Design review of the part shown in the three views and the two pictorial views. Dimensions are in mm from the part's minimum x, y and z. Round coordinates to 2 decimals unless told otherwise and drop trailing zeros. Order: outer loops, then holes, each group sorted by start corner. A loop starts at its lowest first (then second) coordinate and runs counter-clockwise, first axis right, second up. Notation, with made-up numbers: (2.5, 80) - (32.5, 80) arc R10 ccw to (32.5, 91) - close; hole circle Ø10 at (41.5, -20). An arc over 180 degrees is marked (long way). One line per question, with ' | ' between items. Start each with the question number.
Item 1: Add section B-B on x = 18.5. State the section outline as (y, z) points.
Item 2: Add section C-C on y = 10.25. State the section outline as (x, z) points, and give its area (3 significant figures).
Item 3: Add section A-A on z = 11.75. State the section outline as (x, y) points, and give its area (3 significant figures).
Item 4: Insertion check: pin 1 Ø12 at (x, z) = (30, 3.5) entering from +Y; pin 2 Ø0.6 at (y, z) = (1.5, 14.5) entering from +X; pin 3 Ø0.6 at (y, z) = (1, 16.5) entering from -X. Each pin has a flat end and moves straight along its axis. Give the tip position at first contact, or say it passes through.
Item 5: For L1, parallel to X at y = 1, z = 17; L2, parallel to Y at x = 25.5, z = 27; L3, parallel to Y at x = 36.5, z = 11, list the stretches that pass through material, from the lowest coordinate up. Write a range as [from, to].
Item 6: Add section D-D on y = 5. State the section outline as (x, z) points, and give its area (3 significant figures).
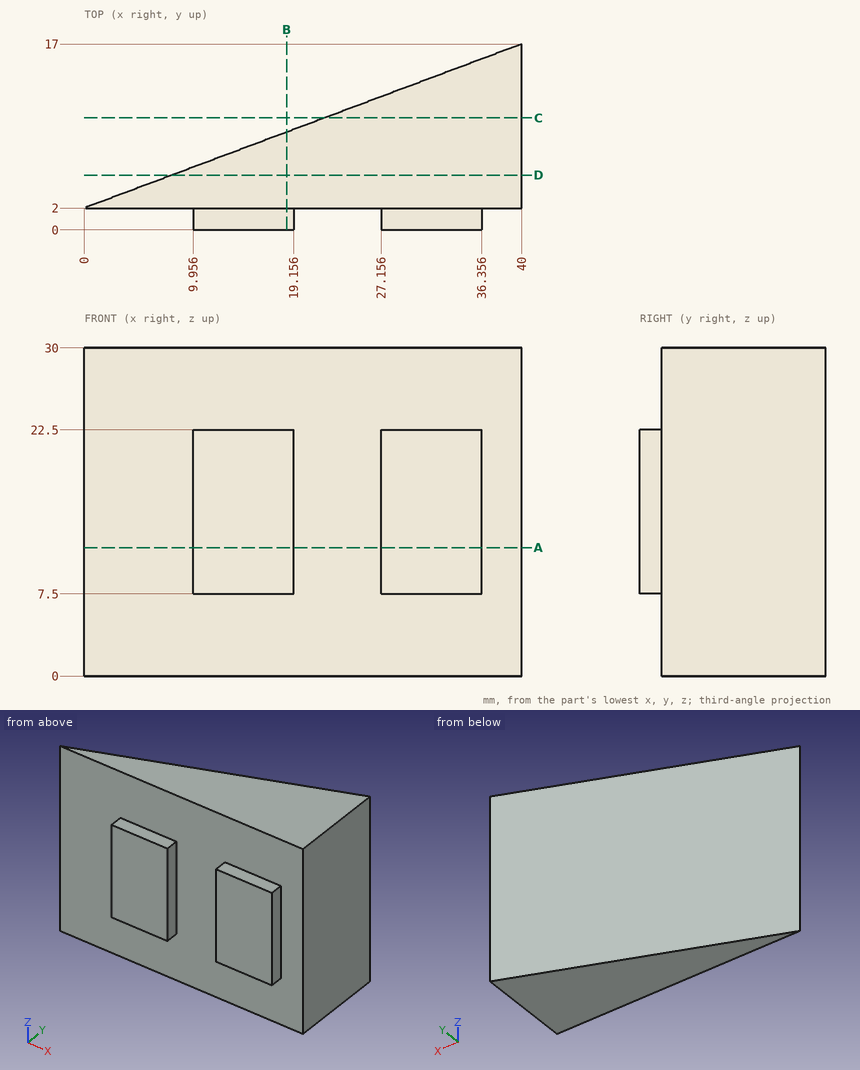
Determined:
1) outline: (0, 7.5) - (2, 7.5) - (2, 0) - (8.94, 0) - (8.94, 30) - (2, 30) - (2, 22.5) - (0, 22.5) - close
2) outline: (22, 0) - (40, 0) - (40, 30) - (22, 30) - close | area: 540 mm2
3) outline: (0, 2) - (9.96, 2) - (9.96, 0) - (19.16, 0) - (19.16, 2) - (27.16, 2) - (27.16, 0) - (36.36, 0) - (36.36, 2) - (40, 2) - (40, 17) - close | area: 337 mm2
4) pin 1: y = 15.5 | pin 2: x = 36.36 | pin 3: x = 9.96
5) L1: [9.96, 19.16], [27.16, 36.36] | L2: [2, 11.56] | L3: [2, 15.69]
6) outline: (8, 0) - (40, 0) - (40, 30) - (8, 30) - close | area: 960 mm2
